Verification items for the finished model (mm, model axes). Face numbers are marked on the shaded views. A direction names the side the tool comes from. Give positions to 0.01 mm unless a question says otherwise; leave off trailing zeros. Loops run counter-clockwise (first coordinate to the right, second up) from the corner with the lowest first, then second, coordinate; pieces in that order, holes last. Notation, with made-up numbers: (-25, 83.25) - (-20, 83.25) arc R11 ccw to (-20, 92.25) - close; hole circle Ø5 at (-19.5, 30.25). An arc over 180 degrees is marked (long way). Answer in a Markdown table with one row per item.
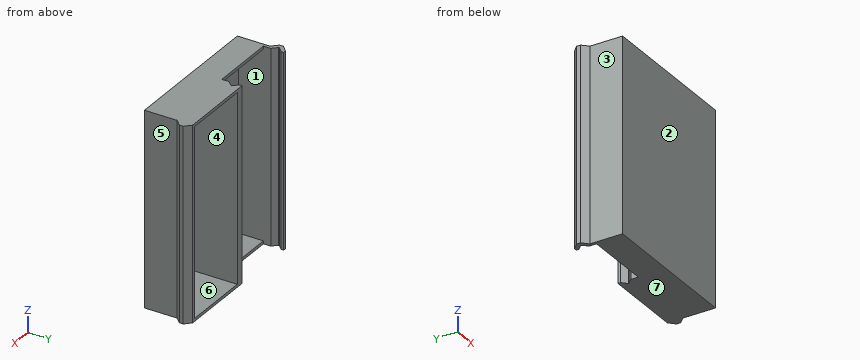
```python
from build123d import *

# Parameters (mm, degrees)
EXTRUDE_1_DEPTH     = 200
SKETCH_2_W          = 148
SKETCH_2_H          = 194
CUT_EXTRUDE_1_DEPTH = 46.779006664
SKETCH_3_W          = 8
SKETCH_3_H          = 194
EXTRUDE_1_2_DEPTH   = 46.779006664
CUT_EXTRUDE_2_DEPTH = 223.186744664


with BuildPart() as part:
    # 草图1 → Extrude 1 (new body)
    with BuildSketch(Plane.XY):
        Polygon((77, 0), (-77, 0), (-77, 33.779006664), (-83, 39.779006664), (-83, 43.779006664), (-77, 49.779006664), (77, 49.779006664), (83, 43.779006664), (83, 39.779006664), (77, 33.779006664), align=None)
    extrude(amount=-EXTRUDE_1_DEPTH)

    # 草图2 → 切除-拉伸1 (cut)
    with BuildSketch(Plane(origin=(0, 49.779006664, 0), x_dir=(1, 0, 0), z_dir=(0, 1, 0))):
        with Locations((0, 100)):
            Rectangle(SKETCH_2_W, SKETCH_2_H)
    extrude(amount=-CUT_EXTRUDE_1_DEPTH, mode=Mode.SUBTRACT)

    # 草图3 → Extrude 1 2 (add)
    with BuildSketch(Plane(origin=(0, 3, 0), x_dir=(1, 0, 0), z_dir=(0, 1, 0))):
        with Locations((-1, 100)):
            Rectangle(SKETCH_3_W, SKETCH_3_H)
    extrude(amount=EXTRUDE_1_2_DEPTH)

    # 草图4 → 切除-拉伸2 (cut, through all)
    with BuildSketch(Plane.XY):
        Polygon((-74, 49.779006664), (-74, 47.122152414), (-79, 42.122152414), (-79, 41.435860913), (-74, 36.435860913), (-74, 28.779006664), (-5, 28.779006664), (-5, 36.435860913), (0, 41.435860913), (0, 42.122152414), (-5, 47.122152414), (-5, 49.779006664), align=None)
    extrude(amount=-CUT_EXTRUDE_2_DEPTH, mode=Mode.SUBTRACT)


solid = part.part
```
Q1. Sectioned sample at A-A (y = 31). Record the cut outline in (x, z).
Completed:
| item | result |
|---|---|
| outline | (-77, -200) - (-74, -200) - (-74, 0) - (-77, 0) - close; (-5, -200) - (77, -200) - (77, 0) - (-5, 0) - close; hole (3, -197) - (74, -197) - (74, -3) - (3, -3) - close |
Q2. Draft check along X on the marked faces 1, 2, 3 and 4. Enter one of: +X half, -X half, draft (parallel to the pull), parting line (faces both ways), or undercut.
Completed:
| item | result |
|---|---|
| face 1 | undercut |
| face 2 | draft |
| face 3 | -X half |
| face 4 | undercut |
Q3. Tool access check on the marked faces 5, 6 and 7. Record the directions out of +Z, -Z, +X, -X, +Y, -Y that give a thin tool (end or side, any length) a straight path to the whole face; none if there is none.
Completed:
| item | result |
|---|---|
| face 5 | +Z, -Z, +X, -Y |
| face 6 | +Y |
| face 7 | -Z, +X, -X, +Y, -Y |
Q4. Go/stop test with flat-tipped pins: P1, Ø12, axis at x = 61.5, y = 7.5, coming from the +Z side; P2, Ø20.5, axis at x = -41.5, z = -107.5, coming from the +Y side; P3, Ø17, axis at y = 15.5, z = -79, coming from the -X side; P4, Ø0.8, axis at y = 48, z = -88, coming from the -X side. Record where each tip stops, or that it passes through.
Completed:
| item | result |
|---|---|
| P1 | z = 0 |
| P2 | y = 3 |
| P3 | x = -77 |
| P4 | x = -79.18 |
Q5. Sectioned sample at C-C (y = 7.5). Record the cut outline in (x, z).
Completed:
| item | result |
|---|---|
| outline | (-77, -200) - (77, -200) - (77, 0) - (-77, 0) - close; hole (-74, -197) - (-5, -197) - (-5, -3) - (-74, -3) - close; hole (3, -197) - (74, -197) - (74, -3) - (3, -3) - close |
Q6. Sectioned sample at D-D (z = -139). Record the cut outline in (x, y), and give its area (3 significant figures).
Completed:
| item | result |
|---|---|
| outline | (-83, 39.78) - (-77, 33.78) - (-77, 0) - (77, 0) - (77, 33.78) - (83, 39.78) - (83, 43.78) - (77, 49.78) - (74, 49.78) - (74, 3) - (3, 3) - (3, 49.78) - (-5, 49.78) - (-5, 47.12) - (0, 42.12) - (0, 41.44) - (-5, 36.44) - (-5, 3) - (-74, 3) - (-74, 36.44) - (-79, 41.44) - (-79, 42.12) - (-74, 47.12) - (-74, 49.78) - (-77, 49.78) - (-83, 43.78) - close |
| area | 1,180 mm^2 |
Q7. Sectioned sample at B-B (x = 30). Record the cut outline in (y, z).
Completed:
| item | result |
|---|---|
| outline | (0, -200) - (49.78, -200) - (49.78, -197) - (3, -197) - (3, -3) - (49.78, -3) - (49.78, 0) - (0, 0) - close |
Q8. Thickness scan on line 1 (X direction, y = 23, z = -182.5); line 2 (Z direction, x = 45, y = 38); line 3 (Y direction, x = 19, z = -12). Record the ranges inside material, lowest first.
Completed:
| item | result |
|---|---|
| line 1 | -77 to -74, -5 to 3, 74 to 77 |
| line 2 | -200 to -197, -3 to 0 |
| line 3 | 0 to 3 |
